```python
from build123d import *

# Parameters (mm, degrees)
F4_DEPTH     = 31.75
F6_DEPTH     = 80.772
F7_W         = 115.0478571653
F7_H         = 280.0295129418
F8_DEPTH     = 80.01
F10_R        = 5.08
F11_R        = 5.08
F12_R        = 1.27
F13_T4_DEPTH = 185.7457951761
F13_T9_DEPTH = 185.7457951761
F15_R        = 18.2048484519
F16_DEPTH    = 25.4


# Not quite as in the source:
# - a fillet or chamfer that OpenCascade refuses, or shapes differently, is made with other operations: its cross-section is extruded or revolved along the edge and cut away or added
# - a feature of the source that left no trace in its solid (it failed there, or was rolled back) is left out


with BuildPart() as f4:
    # F3 (on Right) → F4 (new body, symmetric)
    with BuildSketch(Plane.YZ):
        Polygon((33.4092862904, 0), (34.8578840494, 0), (34.8578840494, 165.3004437685), (51.5383556485, 200.2867460251), (45.9728437156, 202.9402234647), (21.1225822568, 165.3004437685), align=None)
    extrude(amount=F4_DEPTH, both=True)

    # F5 (on Front) → F6 (cut, symmetric)
    with BuildSketch(Plane.XZ):
        Polygon((-36.7620885372, 0), (-2.4731955491, 0), (-9.2842681333, 165.0800704956), (-36.7620885372, 165.0800704956), align=None)
    extrude(amount=F6_DEPTH, both=True, mode=Mode.SUBTRACT)

    # F7 (on Front) → F8 (cut)
    with BuildSketch(Plane.XZ):
        with Locations((57.5239285827, 90.4524587095)):
            Rectangle(F7_W, F7_H)
    extrude(amount=-F8_DEPTH, mode=Mode.SUBTRACT)

    # F9: F4 across face


with BuildPart() as f4_1:
    add(f4.part)
    add(f4.part.mirror(Plane(origin=(0, 31.8435446529, 122.6723093361), x_dir=(0, 1, 0), z_dir=(1, 0, 0))))

    # F10
    f10_edges = [f4_1.edges().sort_by_distance(p)[0] for p in [
        (-9.284268, 27.998423, 165.08007),
        (9.284268, 27.998423, 165.08007),
        (31.75, 27.998423, 165.08007),
        (-31.75, 27.998423, 165.08007),
    ]]
    fillet(f10_edges, radius=F10_R)

    # F11
    f11_edges = [f4_1.edges().sort_by_distance(p)[0] for p in [
        (-31.75, 48.7556, 201.613485),
        (31.75, 48.7556, 201.613485),
    ]]
    fillet(f11_edges, radius=F11_R)

    # F12
    f12_edges = [f4_1.edges().sort_by_distance(p)[0] for p in [
        (-31.75, 33.738898, 184.409914),
    ]]
    fillet(f12_edges, radius=F12_R)

    # F13: fillet of radius 5.08 on 2 edges, made by hand


with BuildPart() as f13_tool2:
    # F13_s3 → F13_t4 (new body)
    with BuildSketch(Plane(origin=(7.1378657639, 0, 173.0005617946), x_dir=(0, 1, 0), z_dir=(-0.0412241322, 0, -0.9991499241))):
        with BuildLine():
            ThreePointArc((29.7778840494, 2.4710931453), (33.3699864978, 0.9831955937), (34.8578840494, -2.6089068547))
            Line((34.8578840494, -2.6089068547), (34.8578840494, 2.4710931453))
            Line((34.8578840494, 2.4710931453), (29.7778840494, 2.4710931453))
        make_face()
    extrude(amount=F13_T4_DEPTH)

    split(bisect_by=Plane(origin=(0, -35.8121563615, 17.0742152946), x_dir=(1, 0, 0), z_dir=(0, 0.902656838, -0.4303610493)), keep=Keep.TOP)


with BuildPart() as f4_2:
    add(f4_1.part)

    # F13_t1: cut F13_tool2
    add(f13_tool2.part, mode=Mode.SUBTRACT)


with BuildPart() as f13_tool7:
    # F13_s8 → F13_t9 (new body)
    with BuildSketch(Plane(origin=(-7.1378657639, 0, 173.0005617946), x_dir=(0, 1, 0), z_dir=(0.0412241322, 0, -0.9991499241))):
        with BuildLine():
            ThreePointArc((29.7778840494, -2.4710931453), (33.3699864978, -0.9831955937), (34.8578840494, 2.6089068547))
            Line((34.8578840494, 2.6089068547), (34.8578840494, -2.4710931453))
            Line((34.8578840494, -2.4710931453), (29.7778840494, -2.4710931453))
        make_face()
    extrude(amount=F13_T9_DEPTH)

    split(bisect_by=Plane(origin=(0, -35.8121563615, 17.0742152946), x_dir=(1, 0, 0), z_dir=(0, 0.902656838, -0.4303610493)), keep=Keep.TOP)


with BuildPart() as f4_3:
    add(f4_2.part)

    # F13_t6: cut F13_tool7
    add(f13_tool7.part, mode=Mode.SUBTRACT)


with BuildPart() as f16:
    # F15 (on line) → F16 (new body)
    with BuildSketch(Plane(origin=(0, -63.794974886, 26.4515642177), x_dir=(-1, 0, 0), z_dir=(0, 0.9237421686, -0.3830148901))):
        with Locations((-38.6807657778, 154.1410535574)):
            Circle(F15_R)
    extrude(amount=F16_DEPTH)


solid = f16.part
```
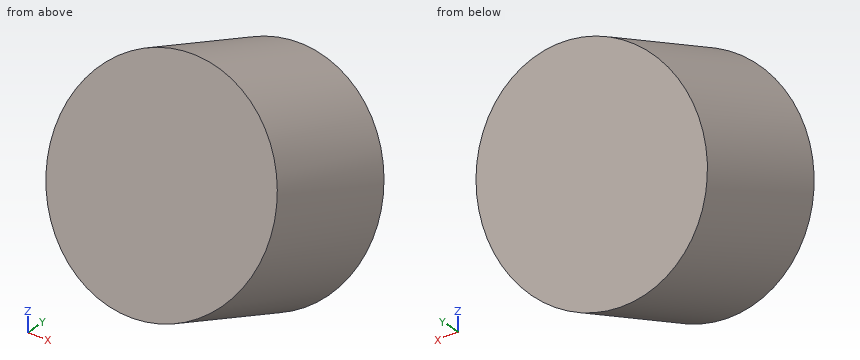
Geometry check sheet. Reference: the model listing, model coordinates, mm. Round coordinates to 2 decimals unless told otherwise and drop trailing zeros. Loops run counter-clockwise (first coordinate to the right, second up) from the corner with the lowest first, then second, coordinate; pieces in that order, holes last. Notation, with made-up numbers: (57, 67.5) - (88, 67.5) arc R12 ccw to (88, 80.5) - close; hole circle Ø11 at (65, 85). An arc over 180 degrees is marked (long way). Write item = value, one per line. Start each with the question number.
1. Depth check by flat-ended pin: pin 1 (12 mm diameter, centred on x = 48.5, y = -6.5, fed in from +Z); pin 2 (4 mm diameter, centred on x = 50.5, y = 1, fed in from +Z); pin 3 (10 mm diameter, centred on y = 15, z = 168, fed in from -X). Enter the tip coordinate at first touch or a pass-through.
2. Thickness scan on line 1 (Z direction, x = 25.5, y = 19.5); line 2 (Z direction, x = 47, y = 24); line 3 (X direction, y = 8.5, z = 173). Record the ranges inside material, lowest first.
3. Section check B-B on x = 25.5. Enter the section's corners in (y, z), then the cut area to 3 significant figures.
4. Section check A-A on x = 43.5. Enter the section's corners in (y, z).
Working result:
q1.pin_1 = 179.1
q1.pin_2 = 183
q1.pin_3 = 20.56
q2.line_1 = 161.02 to 172.37
q2.line_2 = 171.88 to 174.44
q2.line_3 = 22.81 to 54.55
q3.outline = (-9.57, 157.24) - (13.9, 147.51) - (23.52, 170.71) - (0.05, 180.44) - close
q3.area = 638 mm^2
q4.outline = (-11.48, 152.62) - (11.98, 142.89) - (25.43, 175.33) - (1.97, 185.05) - close
